from build123d import *

# Parameters (mm, degrees)
F1_R     = 13.7541
F1_R_2   = 10.6807
F2_DEPTH = 64.008
F3_R     = 13.7541
F3_R_2   = 10.6807
F4_DEPTH = 31.5214
F5_DEPTH = 64.009
F6_DEPTH = 25.4


with BuildPart() as f2:
    # F1 (on offset) → F2 (new body)
    with BuildSketch(Plane.XZ.offset(31.6484)):
        Circle(F1_R)
        Circle(F1_R_2, mode=Mode.SUBTRACT)
    extrude(amount=F2_DEPTH)

    # F3 (on Top) → F4 (join)
    with BuildSketch(Plane.XY):
        with Locations((0, -63.6524)):
            Circle(F3_R)
        with Locations((0, -63.6524)):
            Circle(F3_R_2, mode=Mode.SUBTRACT)
    extrude(amount=-F4_DEPTH)

    # F1 (on offset) → F5 (cut, through all)
    with BuildSketch(Plane.XZ.offset(31.6484)):
        Circle(F1_R_2)
    extrude(amount=F5_DEPTH, mode=Mode.SUBTRACT)

    # F3 (on Top) → F6 (cut)
    with BuildSketch(Plane.XY):
        with Locations((0, -63.6524)):
            Circle(F3_R_2)
    extrude(amount=-F6_DEPTH, mode=Mode.SUBTRACT)


solid = f2.part
CAD build for the part. Positions are in the model's coordinates, mm. A direction names the side the tool comes from. Round coordinates to 2 decimals unless told otherwise and drop trailing zeros. Order: outer loops, then holes, each group sorted by start corner. A loop starts at its lowest first (then second) coordinate and runs counter-clockwise, first axis right, second up. Notation, with made-up numbers: (-19.5, 45.5) -> (11.5, 45.5) arc R31 ccw to (11.5, 76.5) -> close; hole circle Ø3 at (86.5, 88.5). An arc over 180 degrees is marked (long way). Write each question's results on one line, items separated by ' | '.
1. Pull direction Z, two halves, no side cores. Call faces 1 (the face through (7, -72, -31.521)), 2 (the face through (-1.39, -63.2, 10.59)), 3 (the face through (-10.14, -54.36, -19.04)): pulls with the +Z half, pulls with the -Z half, needs draft (parallel to the pull), parting line crosses it, or undercut.
Findings below:
face 1: pulls with the -Z half | face 2: undercut | face 3: needs draft
2. 3-axis set-ups, long thin cutter, end or side, ignore diameter. For faces 4 (the face through (-8.2, -31.648, -7.1)), 5 (the face through (-1.791, -63.204, 13.637)): which of +Z, -Z, +X, -X, +Y, -Y reach the whole face in a straight line?
Findings below:
face 4: +Z, -Z, +X, -X, +Y | face 5: none
3. Flat gauge pins, fed straight in: P1, Ø12, axis at x = 3, z = -26, coming from the -Y side; P2, Ø8, axis at y = -50, z = -14, coming from the -X side; P3, Ø1.5, axis at y = -68.5, z = 5, coming from the +X side. Where does each tip first touch, or does it go through?
Findings below:
P1: stops at y = -77.41 | P2: stops at x = -9.8 | P3: stops at x = 13.08
4. Cut at C-C (y = -48). Give the cut face in (x, z), plus the area to 3 significant figures.
Findings below:
outline: circle Ø27.51 at (0, 0); hole circle Ø21.36 at (0, 0) | area: 236 mm²
5. Cut at B-B (z = -7.5). Give the cut face in (x, y), plus the area to 3 significant figures.
Findings below:
outline: (-11.53, -95.66) -> (-7.6, -95.66) -> (-7.6, -71.15) arc R10.68 cw to (-7.6, -56.15) -> (-7.6, -31.65) -> (-11.53, -31.65) -> (-11.53, -56.15) arc R13.75 ccw to (-11.53, -71.15) -> close; (7.6, -95.66) -> (11.53, -95.66) -> (11.53, -71.15) arc R13.75 ccw to (11.53, -56.15) -> (11.53, -31.65) -> (7.6, -31.65) -> (7.6, -56.15) arc R10.68 cw to (7.6, -71.15) -> close | area: 484 mm²
6. Cut at D-D (x = -8.75). Give the cut face in (y, z).
Findings below:
outline: (-95.66, -10.61) -> (-74.26, -10.61) -> (-74.26, -31.52) -> (-69.78, -31.52) -> (-69.78, -6.12) -> (-95.66, -6.12) -> close; (-95.66, 6.12) -> (-31.65, 6.12) -> (-31.65, 10.61) -> (-95.66, 10.61) -> close; (-57.53, -31.52) -> (-53.04, -31.52) -> (-53.04, -10.61) -> (-31.65, -10.61) -> (-31.65, -6.12) -> (-57.53, -6.12) -> close
7. Cut at A-A (x = 0). Give the cut face in (y, z), plus the area to 3 significant figures.
Findings below:
outline: (-95.66, -13.75) -> (-77.41, -13.75) -> (-77.41, -31.52) -> (-74.33, -31.52) -> (-74.33, -10.68) -> (-95.66, -10.68) -> close; (-95.66, 10.68) -> (-31.65, 10.68) -> (-31.65, 13.75) -> (-95.66, 13.75) -> close; (-52.97, -31.52) -> (-49.9, -31.52) -> (-49.9, -13.75) -> (-31.65, -13.75) -> (-31.65, -10.68) -> (-52.97, -10.68) -> close | area: 437 mm²
8. Wall check: line 1 along X through (y, z) = (-78, 0); line 2 along Y through (x, z) = (0, -25.25); line 3 along Y through (x, z) = (8.5, -14.5) (3 decimals). Give the ranges that are in metal, low to high. Write a range as [from, to].
Findings below:
line 1: x = [-13.75, -10.68], [10.68, 13.75] | line 2: y = [-77.41, -74.33], [-52.97, -49.9] | line 3: y = [-74.466, -70.12], [-57.185, -52.839]
